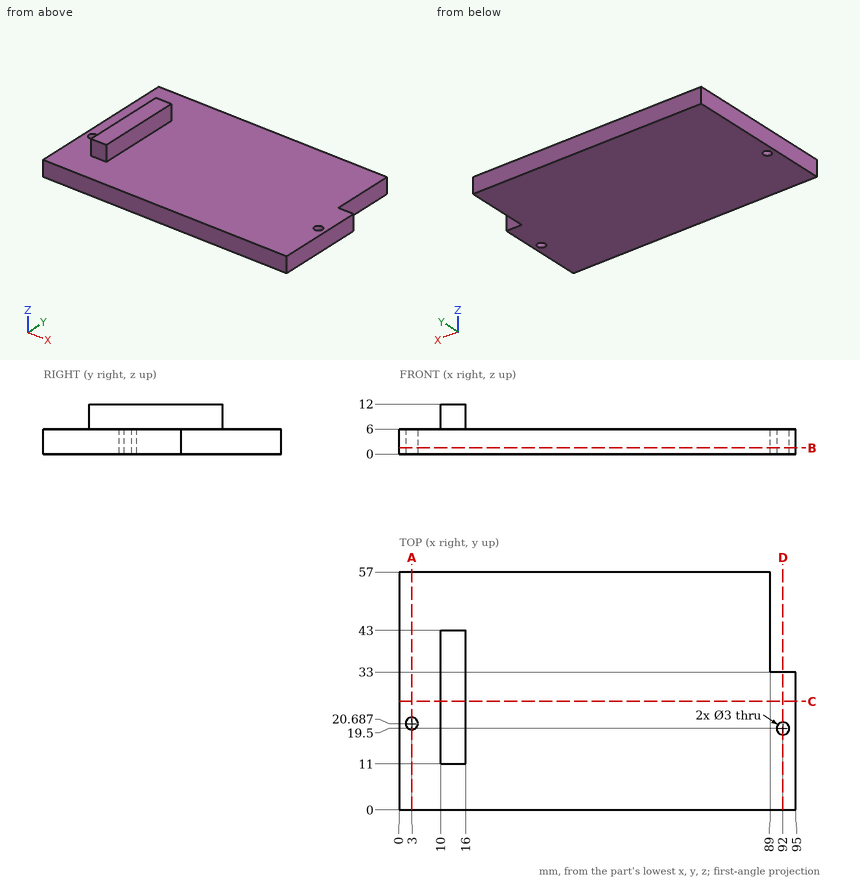
Geometry: see drawing. Coordinates: mm, zero at the bounding-box minimum. Coordinates: 2 decimals unless noted, no trailing zeros. Loops run counter-clockwise (first coordinate to the right, second up) from the corner with the lowest first, then second, coordinate; pieces in that order, holes last. Notation, with made-up numbers: (77, -13) -> (105, -13) arc R26 ccw to (105, 18) -> close; hole circle Ø5 at (4.25, 60.5). An arc over 180 degrees is marked (long way). Write item = value, one per line. Start each with the question number.
Item 1: Cut plane A-A, the plane x = 3. Return loops of the section in (y, z), plus the area to 3 significant figures.
Item 2: Cut plane B-B, the plane z = 1.5. Return loops of the section in (x, y).
Item 3: Cut plane D-D, the plane x = 92. Return loops of the section in (y, z), plus the area to 3 significant figures.
Item 4: Cut plane C-C, the plane y = 26. Return loops of the section in (x, z), plus the area to 3 significant figures.
Item 5: First-contact query: P1, Ø1, axis at y = 34.5, z = 5, coming from the +X side; P2, Ø3.5, axis at x = 3, y = 20.69, coming from the +Z side; P3, Ø3, axis at x = 93, z = 4, coming from the +Y side. Flat tips, straight axial feed; report the tip coordinate or a pass-through.
Item 6: Material intervals for line 1 (Y direction, x = 92, z = 2.8); line 2 (Z direction, x = 29, y = 18.5); line 3 (X direction, y = 39, z = 7), sorted ascending.
Ans:
q1.outline = (0, 0) -> (19.19, 0) -> (19.19, 6) -> (0, 6) -> close; (22.19, 0) -> (57, 0) -> (57, 6) -> (22.19, 6) -> close
q1.area = 324 mm²
q2.outline = (0, 0) -> (95, 0) -> (95, 33) -> (89, 33) -> (89, 57) -> (0, 57) -> close; hole circle Ø3 at (3, 20.69); hole circle Ø3 at (92, 19.5)
q3.outline = (0, 0) -> (18, 0) -> (18, 6) -> (0, 6) -> close; (21, 0) -> (33, 0) -> (33, 6) -> (21, 6) -> close
q3.area = 180 mm²
q4.outline = (0, 0) -> (95, 0) -> (95, 6) -> (16, 6) -> (16, 12) -> (10, 12) -> (10, 6) -> (0, 6) -> close
q4.area = 606 mm²
q5.P1 = 89
q5.P2 = 6
q5.P3 = 33
q6.line_1 = 0 to 18, 21 to 33
q6.line_2 = 0 to 6
q6.line_3 = 10 to 16
